from build123d import *

# Parameters (mm, degrees)
SKETCH_1_W          = 280
SKETCH_1_H          = 90
SKETCH_1_R          = 1.5
SKETCH_1_W_2        = 15
SKETCH_1_H_2        = 4
EXTRUDE_1_DEPTH     = 4
SKETCH_2_W          = 4
SKETCH_2_H          = 30
SKETCH_2_R          = 1.4
SKETCH_2_W_2        = 20
SKETCH_2_H_2        = 4
SKETCH_2_W_3        = 40
EXTRUDE_7_DEPTH     = 4
CUT_EXTRUDE_1_DEPTH = 153.161098839


with BuildPart() as part:
    # Эскиз1 → Бобышка-Вытянуть1 (new body)
    with BuildSketch(Plane.XY):
        Rectangle(SKETCH_1_W, SKETCH_1_H)
        with Locations((11.25, 6.5)):
            Circle(SKETCH_1_R, mode=Mode.SUBTRACT)
        with Locations((-11.25, 6.5)):
            Circle(SKETCH_1_R, mode=Mode.SUBTRACT)
        with Locations((-11.25, -39.5)):
            Circle(SKETCH_1_R, mode=Mode.SUBTRACT)
        with Locations((11.25, -39.5)):
            Circle(SKETCH_1_R, mode=Mode.SUBTRACT)
        with Locations((0, -39.5)):
            Rectangle(SKETCH_1_W_2, SKETCH_1_H_2, mode=Mode.SUBTRACT)
        with Locations((0, 6.5)):
            Rectangle(SKETCH_1_W_2, SKETCH_1_H_2, mode=Mode.SUBTRACT)
    extrude(amount=EXTRUDE_1_DEPTH)

    # Эскиз2 → Бобышка-Вытянуть7 (add, through all)
    # profile 1 of 7: a face of its own
    with BuildSketch(Plane.XY):
        with Locations((-142, 0)):
            Rectangle(SKETCH_2_W, SKETCH_2_H)
        with Locations((-141.75, 0)):
            Circle(SKETCH_2_R, mode=Mode.SUBTRACT)
    # profile 2 of 7: a face of its own
    with BuildSketch(Plane.XY):
        with Locations((-130, 47)):
            Rectangle(SKETCH_2_W_2, SKETCH_2_H_2)
        with Locations((-130, 46.75)):
            Circle(SKETCH_2_R, mode=Mode.SUBTRACT)
    # profile 3 of 7: a face of its own
    with BuildSketch(Plane.XY):
        with Locations((-0.75, 47)):
            Rectangle(SKETCH_2_W_3, SKETCH_2_H_2)
        with Locations((9.25, 46.75)):
            Circle(SKETCH_2_R, mode=Mode.SUBTRACT)
        with Locations((-10.75, 46.75)):
            Circle(SKETCH_2_R, mode=Mode.SUBTRACT)
    # profile 4 of 7: a face of its own
    with BuildSketch(Plane.XY):
        with Locations((130, 47)):
            Rectangle(SKETCH_2_W_2, SKETCH_2_H_2)
        with Locations((130, 46.75)):
            Circle(SKETCH_2_R, mode=Mode.SUBTRACT)
    # profile 5 of 7: a face of its own
    with BuildSketch(Plane.XY):
        with Locations((142, 0)):
            Rectangle(SKETCH_2_W, SKETCH_2_H)
        with Locations((141.75, 0)):
            Circle(SKETCH_2_R, mode=Mode.SUBTRACT)
    # profile 6 of 7: a face of its own
    with BuildSketch(Plane.XY):
        with Locations((-67.75, 47)):
            Rectangle(SKETCH_2_W_2, SKETCH_2_H_2)
        with Locations((-67.75, 46.75)):
            Circle(SKETCH_2_R, mode=Mode.SUBTRACT)
    # profile 7 of 7: a face of its own
    with BuildSketch(Plane.XY):
        with Locations((67.75, 47)):
            Rectangle(SKETCH_2_W_2, SKETCH_2_H_2)
        with Locations((67.75, 46.75)):
            Circle(SKETCH_2_R, mode=Mode.SUBTRACT)
    extrude(amount=EXTRUDE_7_DEPTH)

    # Эскиз3 → Вырез-Вытянуть1 (cut, through all)
    with BuildSketch(Plane.XY.offset(4)):
        Polygon((97.375, 42), (96.325, 42), (96.325, 40), (97.375, 40), (97.375, 39), (100.375, 39), (100.375, 40), (101.425, 40), (101.425, 42), (100.375, 42), (100.375, 45), (97.375, 45), align=None)
        Polygon((-97.375, 45), (-100.375, 45), (-100.375, 42), (-101.425, 42), (-101.425, 40), (-100.375, 40), (-100.375, 39), (-97.375, 39), (-97.375, 40), (-96.325, 40), (-96.325, 42), (-97.375, 42), align=None)
        Polygon((-137, 31.5), (-140, 31.5), (-140, 28.5), (-137, 28.5), (-137, 27.45), (-135, 27.45), (-135, 28.5), (-134, 28.5), (-134, 31.5), (-135, 31.5), (-135, 32.55), (-137, 32.55), align=None)
        Polygon((-137, -32.55), (-135, -32.55), (-135, -31.5), (-134, -31.5), (-134, -28.5), (-135, -28.5), (-135, -27.45), (-137, -27.45), (-137, -28.5), (-140, -28.5), (-140, -31.5), (-137, -31.5), align=None)
        Polygon((137, -31.5), (140, -31.5), (140, -28.5), (137, -28.5), (137, -27.45), (135, -27.45), (135, -28.5), (134, -28.5), (134, -31.5), (135, -31.5), (135, -32.55), (137, -32.55), align=None)
        Polygon((137, 32.55), (135, 32.55), (135, 31.5), (134, 31.5), (134, 28.5), (135, 28.5), (135, 27.45), (137, 27.45), (137, 28.5), (140, 28.5), (140, 31.5), (137, 31.5), align=None)
    extrude(amount=-CUT_EXTRUDE_1_DEPTH, mode=Mode.SUBTRACT)


solid = part.part
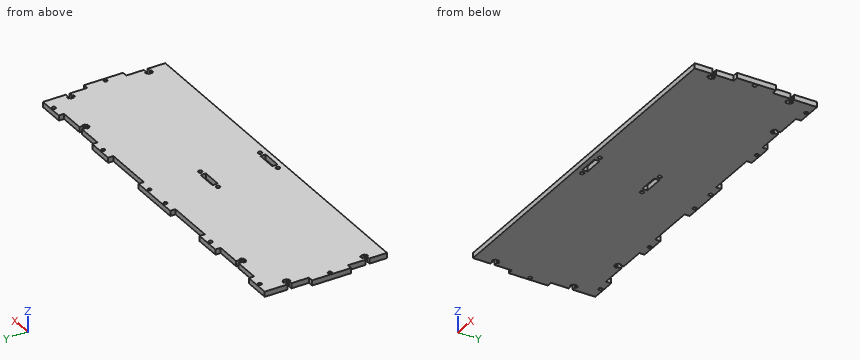
Work out the finished part from the listing and answer in its coordinate system (mm). Round coordinates to 2 decimals unless told otherwise and drop trailing zeros. Loops run counter-clockwise (first coordinate to the right, second up) from the corner with the lowest first, then second, coordinate; pieces in that order, holes last. Notation, with made-up numbers: (-39.5, 85.25) - (-22.5, 85.25) arc R16 cw to (-22.5, 97.25) - close; hole circle Ø5 at (47.5, -23.5). An arc over 180 degrees is marked (long way). One line per item, written item: value.
Q1. Find section A-A on z = 2.35. State how many separate pieces and enclosed holes the cut face has, and give its area (3 significant figures).
Check values:
separate pieces: 1
enclosed holes: 14
area: 25,600 mm2
Q2. Each of these flat-tipped pins is pushed along its axis until it touches: pin 1 Ø2 at (y, z) = (48, 1.5) entering from +X; pin 2 Ø2 at (x, y) = (-10.75, 46.75) entering from +Z; pin 3 Ø3 at (x, y) = (-111.5, -8) entering from -Z; pin 4 Ø1.2 at (y, z) = (-22.5, 2.5) entering from -X. Where does it stop, or does it pass through?
Check values:
pin 1: x = 140
pin 2: through
pin 3: z = 0
pin 4: x = -140
Q3. Find section B-B on x = -88. Give the vertices of the cut face in (y, z), and give its area (3 significant figures).
Check values:
outline: (-45, 0) - (45, 0) - (45, 4) - (-45, 4) - close
area: 360 mm2
Q4. Straight lines are drawn through the part: probe 1 along X at (y, z) = (41.5, 1.55) (3 decimals); probe 2 along Y at (x, z) = (141.75, 1.75); probe 3 along Y at (x, z) = (-130, 1.3). For each, find the intervals that lie inside material, in ascending order.
Check values:
probe 1: -140 to -101.425, -96.325 to 96.325, 101.425 to 140
probe 2: -15 to -1.4, 1.4 to 15
probe 3: -45 to 45.35, 48.15 to 49
Q5. Find section C-C on y = 36. Give the vertices of the cut face in (x, z), and give its area (3 significant figures).
Check values:
outline: (-140, 0) - (140, 0) - (140, 4) - (-140, 4) - close
area: 1,120 mm2
